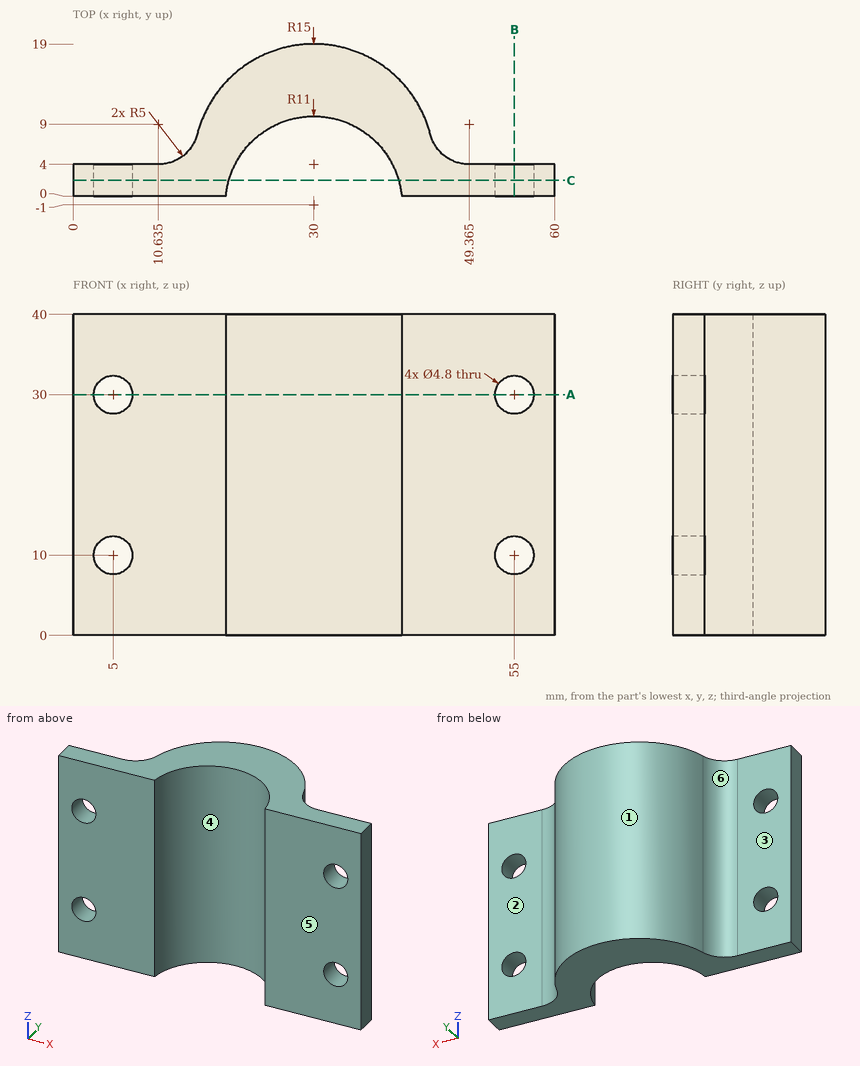
Drawing for the job (mm, zero at the part's lowest x, y, z). A direction names the side the tool comes from. Coordinates: 2 decimals unless noted, no trailing zeros. Write each loop counter-clockwise with the first axis right and the second up, starting at its lowest first coordinate (ties: lowest second). Pieces come first, ordered by that corner, then holes. Notation, with made-up numbers: (-35, 72.5) - (3, 72.5) arc R20 ccw to (3, 103.5) - close; hole circle Ø9 at (20.5, -28). An arc over 180 degrees is marked (long way). Write each question's results on one line, items separated by ' | '. Start each with the question number.
1) Cut at B-B (x = 55). Write the cut outline in (y, z), then the cut area to 3 significant figures.
2) Cut at A-A (z = 30). Count the separate pieces of the cut face and the enclosed holes in it, then the cut area to 3 significant figures.
3) Mould opens along X. For the marked faces 4, 5 and 6 say: pulls with the +X half, pulls with the -X half, needs draft (parallel to the pull), parting line crosses it, or undercut.
4) Probe line 1 along Z through (x, y) = (5, 2.4); line 2 along X through (y, z) = (0.8, 30); line 3 along Y through (x, z) = (53.5, 16.5). List the from-to ranges inside material, lowest first. Write a range as from..to.
5) 3-axis set-ups, long thin cutter, end or side, ignore diameter. For the marked faces 1, 2 and 3: which of +Z, -Z, +X, -X, +Y, -Y reach the whole face in a straight line?
6) Cut at C-C (y = 2). Write the cut outline in (x, z).
7) Flat gauge pins, fed straight in: P1, Ø6, axis at x = 15, z = 4.5, coming from the +Y side; P2, Ø1.5, axis at x = 42.5, z = 28.5, coming from the +Y side; P3, Ø5.5, axis at x = 55.5, z = 13, coming from the +Y side. Where does each tip first touch, or does it go through?
Returned:
1) outline: (0, 0) - (4, 0) - (4, 7.6) - (0, 7.6) - close; (0, 12.4) - (4, 12.4) - (4, 27.6) - (0, 27.6) - close; (0, 32.4) - (4, 32.4) - (4, 40) - (0, 40) - close | area: 122 mm^2
2) separate pieces: 3 | enclosed holes: 0 | area: 394 mm^2
3) face 4: undercut | face 5: needs draft | face 6: pulls with the -X half
4) line 1: 0..7.6, 12.4..27.6, 32.4..40 | line 2: 0..2.6, 7.4..19.15, 40.85..52.6, 57.4..60 | line 3: 0..4
5) face 1: +Z, -Z, +Y | face 2: +Z, -Z, +X, +Y | face 3: +Z, -Z, -X, +Y
6) outline: (0, 0) - (19.42, 0) - (19.42, 40) - (0, 40) - close; (40.58, 0) - (60, 0) - (60, 40) - (40.58, 40) - close; hole circle Ø4.8 at (5, 10); hole circle Ø4.8 at (5, 30); hole circle Ø4.8 at (55, 10); hole circle Ø4.8 at (55, 30)
7) P1: y = 13 | P2: y = 13.32 | P3: y = 4
